from build123d import *

# Parameters (mm, degrees)
SKETCH1_W                = 418.07892
SKETCH1_H                = 415.925
BOSS_EXTRUDE1_DEPTH      = 12.7
SKETCH2_W                = 418.07892
SKETCH2_H                = 79.68996
BOSS_EXTRUDE2_DEPTH      = 12.7
SKETCH3_W                = 418.07892
SKETCH3_H                = 28.376126504
BOSS_EXTRUDE3_DEPTH      = 12.7
BOSS_EXTRUDE4_DEPTH      = 12.7
CHAMFER1_SIZE            = 304.8
CHAMFER1_SIZE_2          = 19.05
SKETCH5_W                = 12.7
SKETCH5_H                = 15.453987587
CUT_EXTRUDE1_DEPTH       = 5568.603780331
F_5_16_CLEARANCE_HOLE1_D = 8.72998
HOLE1_D                  = 3.175
HOLE1_DEPTH              = 50.8
HOLE1_CSINK_D            = 10.16
HOLE1_CSINK_ANGLE        = 82
HOLE1_TIP                = 0.953866233


with BuildPart() as part:
    # Sketch1 → Boss-Extrude1 (new body)
    with BuildSketch(Plane.XY):
        with Locations((0, -5261.217030575)):
            Rectangle(SKETCH1_W, SKETCH1_H)
    extrude(amount=BOSS_EXTRUDE1_DEPTH)

    # Sketch2 → Boss-Extrude2 (add, through all)
    with BuildSketch(Plane(origin=(0, 0, 0), x_dir=(-1, 0, 0), z_dir=(0, 0, -1))):
        with Locations((0, -5509.024510575)):
            Rectangle(SKETCH2_W, SKETCH2_H)
    extrude(amount=-BOSS_EXTRUDE2_DEPTH)

    # Sketch3 → Boss-Extrude3 (add, through all)
    with BuildSketch(Plane(origin=(0, 0, 0), x_dir=(-1, 0, 0), z_dir=(0, 0, -1))):
        with Locations((0, -5039.066467323)):
            Rectangle(SKETCH3_W, SKETCH3_H)
    extrude(amount=-BOSS_EXTRUDE3_DEPTH)

    # Sketch4 → Boss-Extrude4 (add, through all)
    with BuildSketch(Plane(origin=(0, 0, 0), x_dir=(-1, 0, 0), z_dir=(0, 0, -1))):
        Polygon((209.038766336, -5447.352766987), (228.088766336, -5447.352766987), (228.088766336, -5548.869490575), (209.03946, -5548.869490575), align=None)
        Polygon((-209.03946, -5548.869490575), (-209.038766336, -5447.352766987), (-228.088766336, -5447.352766987), (-228.088766336, -5548.869490575), align=None)
    extrude(amount=-BOSS_EXTRUDE4_DEPTH)

    # Chamfer1
    # the kernel refuses this chamfer: 304.8, 19.05 mm, written as the material it adds along each edge
    with BuildSketch(Plane(origin=(-209.03946, -5447.352766987, 0), x_dir=(0.002399337658707147, 0.9999971215852571, 0), z_dir=(0, 0, 1))) as chamfer1_piece_1_section:
        Polygon((CHAMFER1_SIZE * 0.999997121585, CHAMFER1_SIZE * 0.00239933765871), (-CHAMFER1_SIZE_2 * 0.00239933765871, CHAMFER1_SIZE_2 * 0.999997121585), (0, 0), align=None)
    chamfer1_piece_1 = extrude(amount=12.7, mode=Mode.PRIVATE)
    chamfer1_piece_1 = split(chamfer1_piece_1, bisect_by=Plane(origin=(-228.088766336, -5325.682018196, 6.35), z_dir=(1, 0, 0)), keep=Keep.TOP, mode=Mode.PRIVATE)
    add(chamfer1_piece_1)
    with BuildSketch(Plane(origin=(209.03946, -5447.352766987, 0), x_dir=(0.8520963193143735, -0.5233850041899339, 0), z_dir=(0, 0, 1))) as chamfer1_piece_2_section:
        Polygon((CHAMFER1_SIZE_2 * 0.852096319314, CHAMFER1_SIZE_2 * 0.52338500419), (-CHAMFER1_SIZE * 0.52338500419, CHAMFER1_SIZE * 0.852096319314), (0, 0), align=None)
    chamfer1_piece_2 = extrude(amount=12.7, mode=Mode.PRIVATE)
    chamfer1_piece_2 = split(chamfer1_piece_2, bisect_by=Plane(origin=(228.088766336, -5325.682018196, 6.35), z_dir=(-1, 0, 0)), keep=Keep.TOP, mode=Mode.PRIVATE)
    add(chamfer1_piece_2)

    # Sketch5 → Cut-Extrude1 (cut, through all)
    with BuildSketch(Plane(origin=(228.088766336, 0, 0), x_dir=(0, 0, -1), z_dir=(1, 0, 0))):
        with Locations((-6.35, -5541.142496782)):
            Rectangle(SKETCH5_W, SKETCH5_H)
    extrude(amount=-CUT_EXTRUDE1_DEPTH, mode=Mode.SUBTRACT)

    # 5/16 Clearance Hole1 (through all)
    with Locations(Plane(origin=(0, 0, 0), x_dir=(-1, 0, 0), z_dir=(0, 0, -1))):
        with Locations((138.550999994, -5387.96381451), (-138.550999994, -5387.96381451), (-138.550999994, -5164.31681451), (138.550999994, -5164.31681451)):
            Hole(F_5_16_CLEARANCE_HOLE1_D / 2)

    # Hole1
    with Locations(Plane(origin=(0, -5562.870276207, -19.05), x_dir=(-1, 0, 0), z_dir=(0, 0, -1))):
        with Locations((218.563766336, 102.817509219), (218.563766336, 48.504773219), (202.68946, 123.306744588), (202.68946, 317.949308361), (202.68946, 518.941872135), (88.38946, 518.941872135), (88.38946, 317.949308361), (88.38946, 123.306744588), (104.263766336, 216.849631358), (104.263766336, 132.677202288), (104.263766336, 48.504773219), (-104.263766336, 48.504773219), (-104.263766336, 132.677202288), (-104.263766336, 216.849631358), (-88.38946, 123.306744588), (-88.38946, 317.949308361), (-88.38946, 518.941872135), (-202.68946, 518.941872135), (-202.68946, 317.949308361), (-202.68946, 123.306744588), (-218.563766336, 48.504773219), (-218.563766336, 102.817509219)):
            CounterSinkHole(HOLE1_D / 2, HOLE1_CSINK_D / 2, depth=HOLE1_DEPTH, counter_sink_angle=HOLE1_CSINK_ANGLE)
            with Locations((0, 0, -(HOLE1_DEPTH + HOLE1_TIP / 2))):  # 118° drill point
                Cone(0, HOLE1_D / 2, HOLE1_TIP, mode=Mode.SUBTRACT)


solid = part.part
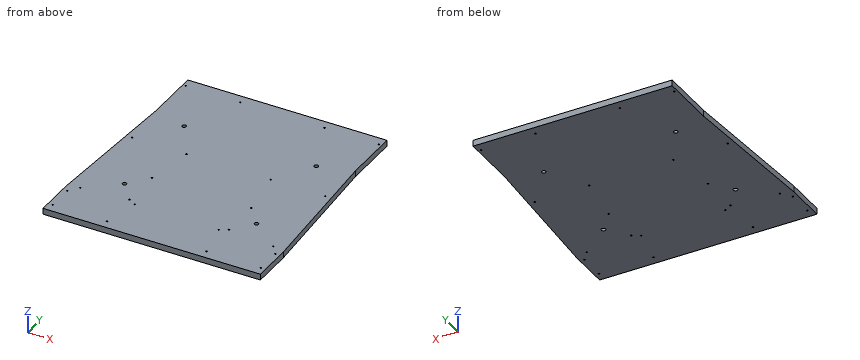
Here's how the part is built. I have some questions about the finished solid (model axes, mm). Round coordinates to 2 decimals unless told otherwise and drop trailing zeros. Loops run counter-clockwise (first coordinate to the right, second up) from the corner with the lowest first, then second, coordinate; pieces in that order, holes last.
1. For P1, Ø6, axis at y = -5158.5, z = 5.5, coming from the -X side; P2, Ø1, axis at y = -5280, z = 11, coming from the -X side, each with a flat end and sliding along its axis, tell me the tip position at first contact or that it passes through.
Answer list:
P1: stops at x = -210.22
P2: stops at x = -217.66
2. If we section it at C-C on y = -5204: Write out the boundary of the cut face in (x, z), plus the area to 3 significant figures.
Answer list:
outline: (-212.88, 0) - (212.88, 0) - (212.88, 12.7) - (-212.88, 12.7) - close
area: 5,410 mm2
3. If we section it at A-A on z = 4: Count the separate pieces of the cut face and the enclosed holes in it, plus the area to 3 significant figures.
Answer list:
separate pieces: 1
enclosed holes: 26
area: 221,000 mm2
4. If we section it at B-B on y = -5106.5: Write out the boundary of the cut face in (x, z), plus the area to 3 significant figures.
Answer list:
outline: (-209.04, 0) - (209.04, 0) - (209.04, 12.7) - (-209.04, 12.7) - close
area: 5,310 mm2
5. If I drill on line 1 along Y through (x, z) = (137, 2); line 2 along X through (y, z) = (-5089, 9); line 3 along X through (y, z) = (-5337, 2.5), over which ranges is the centre line in solid material (lowest first)?
Answer list:
line 1: y = -5533.42 to -5392.04, -5383.88 to -5168.4, -5160.24 to -5024.88
line 2: x = -209.04 to 209.04
line 3: x = -221.19 to 221.19
